Autodesk Fusion 360 part; units mm, degrees
sketch "Sketch1" plane through (0, 0, 0) normal (0, 0, 1) x (1, 0, 0)
  circle A0 centre (0, 0) radius 3.55
  dimension "d1" = 7.1
extrude "Extrude1" add sketch "Sketch1" along normal blind 14
hole "Hole1" at (0, 0, 14) direction (0, 0, -1) diameter 4.7 depth 5 tip angle 180
hole "Hole2" at (0, 0, 0) direction (0, 0, 1) diameter 4.7 depth 5 tip angle 180
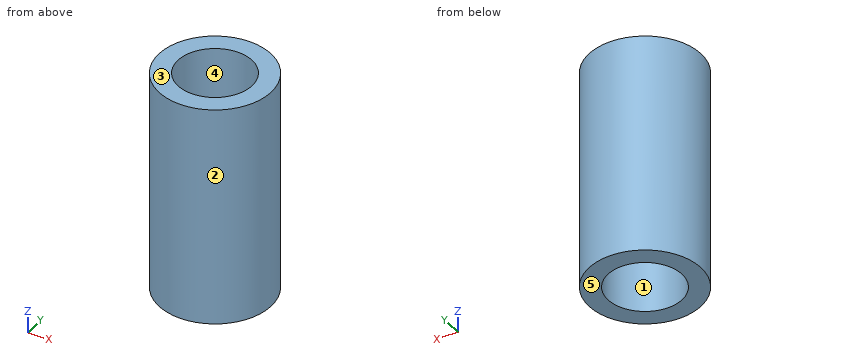
Build history of the part. All positions in model axes, mm. Face numbers are marked on the shaded views. A direction names the side the tool comes from. Round coordinates to 2 decimals unless told otherwise and drop trailing zeros. Write each loop counter-clockwise with the first axis right and the second up, starting at its lowest first coordinate (ties: lowest second). Pieces come first, ordered by that corner, then holes.
1) Drill centre lines: probe 1 along Y at (x, z) = (0, 11.75); probe 2 along Y at (x, z) = (-1.5, 4); probe 3 along Z at (x, y) = (0.75, 1.25). Where is each one in solid material? Low to high.
2) Band-saw the part on D-D, the plane z = 8.5. List the corners of the cut face in (x, y).
3) Band-saw the part on C-C, the plane z = 1. List the corners of the cut face in (x, y), and give its area (3 significant figures).
4) Mould opens along Y. For the marked faces 1, 2 and 3 say: +Y half, -Y half, draft (parallel to the pull), parting line (faces both ways), or undercut.
5) Pin check, flat tip, straight feed: pin 1 (3 mm diameter, centred on x = 0, y = 0, fed in from +Z). Stop position of the tip, or through.
6) 3-axis set-ups, long thin cutter, end or side, ignore diameter. For the marked faces 4 and 5: which of +Z, -Z, +X, -X, +Y, -Y reach the whole face in a straight line?
7) Band-saw the part on A-A, the plane x = 0. List the corners of the cut face in (y, z).
Ans:
1. probe 1: y = -3.55 to -2.35, 2.35 to 3.55
1. probe 2: y = -3.22 to -1.81, 1.81 to 3.22
1. probe 3: z = 5 to 9
2. outline: circle Ø7.1 at (0, 0)
3. outline: circle Ø7.1 at (0, 0); hole circle Ø4.7 at (0, 0)
3. area: 22.2 mm2
4. face 1: undercut
4. face 2: parting line
4. face 3: draft
5. pin 1: stops at z = 9
6. face 4: +Z
6. face 5: -Z, +X, -X, +Y, -Y
7. outline: (-3.55, 0) - (-2.35, 0) - (-2.35, 5) - (2.35, 5) - (2.35, 0) - (3.55, 0) - (3.55, 14) - (2.35, 14) - (2.35, 9) - (-2.35, 9) - (-2.35, 14) - (-3.55, 14) - close
